Autodesk Fusion 360 part; units mm, degrees
sketch "草图1" plane through (0, 0, 0) normal (0, 0, 1) x (1, 0, 0)
  line L0 (-9.0514, 8.5015) -> (8.9486, 8.5015)
  line L1 (8.9486, 8.5015) -> (8.9486, -9.4985)
  line L2 (8.9486, -9.4985) -> (-9.0514, -9.4985)
  line L3 (-9.0514, -9.4985) -> (-9.0514, 8.5015)
  dimension "d3" = 18
  dimension "d4" = 18
extrude "拉伸1" add sketch "草图1" along normal blind 3
sketch "草图2" plane through (0, 0, 0) normal (0, 0, 1) x (1, 0, 0)
  line L0 (-2.5482, 2.0089) -> (2.4518, 2.0089)
  line L1 (2.4518, 2.0089) -> (2.4518, -2.9911)
  line L2 (2.4518, -2.9911) -> (-2.5482, -2.9911)
  line L3 (-2.5482, -2.9911) -> (-2.5482, 2.0089)
  dimension "d7" = 5
  dimension "d8" = 5
extrude "拉伸2" add sketch "草图2" against normal blind 3
Here's how the part is built. I have some questions about the finished solid (model axes, mm). A direction names the side the tool comes from. Coordinates: 2 decimals unless noted, no trailing zeros. Order: outer loops, then holes, each group sorted by start corner. A loop starts at its lowest first (then second) coordinate and runs counter-clockwise, first axis right, second up. Notation, with made-up numbers: (21.25, -4.5) -> (37.25, -4.5) arc R13 ccw to (37.25, 7.5) -> close; hole circle Ø10 at (-37.75, 6). An arc over 180 degrees is marked (long way). Return JSON: item names as keys, results as strings.
1) If we section it at A-A on x = 0.5: List the corners of the cut face in (y, z) for me.
Conclusion:
{"outline": "(-9.5, 0) -> (-2.99, 0) -> (-2.99, -3) -> (2.01, -3) -> (2.01, 0) -> (8.5, 0) -> (8.5, 3) -> (-9.5, 3) -> close"}
2) I'm going to push flat-ended pins straight in: P1, Ø3, axis at x = 2.5, y = 5, coming from the -Z side; P2, Ø1.5, axis at x = -1.5, z = -1, coming from the +Y side; P3, Ø2.5, axis at y = -1, z = -2, coming from the +X side. Where does each tip first touch, or does it pass through?
Conclusion:
{"P1": "stops at z = 0", "P2": "stops at y = 2.01", "P3": "stops at x = 2.45"}
3) If I drill on probe 1 along Z at (x, y) = (-4.5, 0); probe 2 along X at (y, z) = (1.5, -0.6); probe 3 along Y at (x, z) = (-1, -0.85), over which ranges is the centre line in solid material (lowest first)?
Conclusion:
{"probe 1": "z = 0 to 3", "probe 2": "x = -2.55 to 2.45", "probe 3": "y = -2.99 to 2.01"}
4) If we section it at B-B on z = -1.9: List the corners of the cut face in (x, y) for me.
Conclusion:
{"outline": "(-2.55, -2.99) -> (2.45, -2.99) -> (2.45, 2.01) -> (-2.55, 2.01) -> close"}
5) If we section it at C-C on y = -4.75: List the corners of the cut face in (x, z) for me, plus the area to 3 significant figures.
Conclusion:
{"outline": "(-9.05, 0) -> (8.95, 0) -> (8.95, 3) -> (-9.05, 3) -> close", "area": "54.0 mm²"}
6) On a 3-axis mill with a long thin cutter (end or side, diameter ignored), from which of +Z, -Z, +X, -X, +Y, -Y can I reach the whole of each face in a straight line? I mean faces 1 (the flat face through (2.452, 0, -1)), 2 (the flat face through (-2.548, -1, -1)), 3 (the flat face through (0, 2.009, -1)). Say none if no direction works.
Conclusion:
{"face 1": "-Z, +X, +Y, -Y", "face 2": "-Z, -X, +Y, -Y", "face 3": "-Z, +X, -X, +Y"}
